Part model, mm, in its own coordinate system. Coordinates: 2 decimals unless noted, no trailing zeros. Order: outer loops, then holes, each group sorted by start corner. A loop starts at its lowest first (then second) coordinate and runs counter-clockwise, first axis right, second up.
Autodesk Inventor part; units mm, degrees
ref_plane "工作平面1" through (10, 22, 0) normal (-0.3882, -0.6516, -0.6516) x (0.8591, 0, -0.5118)
ref_plane "YZ Plane" through (0, 0, 0) normal (1, 0, 0) x (0, 1, 0)
ref_plane "XZ Plane" through (0, 0, 0) normal (0, 1, 0) x (-1, 0, 0)
sketch "草圖1" plane through (0, 0, 0) normal (0, 1, 0) x (-1, 0, 0)
  line L0 (0, 0) -> (-57, 0)
  line L1 (-57, 0) -> (-57, -38)
  line L2 (-57, -38) -> (0, -38)
  line L3 (0, -38) -> (0, 0)
  dimension "d0" = 57
  dimension "d1" = 38
extrude "擠出1" add sketch "草圖1" along normal mid plane 44
sketch "草圖2" plane through (0, 22, 0) normal (0, 1, 0) x (1, 0, 0)
  line L0 (0, 0) -> (57, 0)
  line L1 (10, 0) -> (57, 8)
  line L2 (57, 0) -> (57, 38)
  dimension "d4" = 10
  dimension "d5" = 30
extrude "擠出2" cut sketch "草圖2" against normal blind 60
sketch "草圖3" plane through (57, -22, -38) normal (1, 0, 0) x (0, 0, -1)
  line L0 (-30, 24) -> (-10, 44)
  line L1 (0, 44) -> (-38, 44)
  line L2 (-30, 44) -> (-30, 0)
  point P0 (-38, 22)
  point P1 (-30, 2)
  dimension "d8" = 20
  dimension "d9" = 20
ref_plane "工作平面1" through (10, 22, 0) normal (-0.3882, -0.6516, -0.6516) x (0.8591, 0, -0.5118)
sketch "草圖4" plane through (10, 22, 0) normal (-0.3882, -0.6516, -0.6516) x (0.8591, 0, -0.5118)
  line L0 (-15.1543, -12.3218) -> (93.717, -12.3218)
  line L1 (93.717, -12.3218) -> (93.717, 28.8166)
  line L2 (93.717, 28.8166) -> (-15.1543, 28.8166)
  line L3 (-15.1543, 28.8166) -> (-15.1543, -12.3218)
  point P0 (-8.591, 13.3523)
extrude "擠出3" cut sketch "草圖4" against normal blind 40
mirror "鏡射1" about plane through (0, 0, 0) normal (0, 1, 0) of "擠出3"
properties part number "52"
(1) Slice it at B-B, the plane x = 19. Give the cut face in (y, z).
(2) Drop flat-ended pins along their axis: pin 1 (12 mm diameter, centred on x = 28, y = -10, fed in from +Z); pin 2 (3 mm diameter, centred on x = 37, y = -5.5, fed in from +Z); pin 3 (1 mm diameter, centred on x = 32, z = -10, fed in from +Y). Give the stop position or say it passes through.
(3) Slice it at C-C, the plane z = -4.5. Give the cut face in (x, y), then the cut area to 3 significant figures.
(4) Slice it at A-A, the plane y = 1. Give the cut face in (x, z), then the cut area to 3 significant figures.
(5) Probe line 1 (Z direction, x = 53.5, y = 5.5); line 2 (X direction, y = 20.5, z = -24.5); line 3 (Z direction, x = 38, y = 13.5). List the from-to ranges inside material, lowest first.
Here are the results:
1. outline: (-22, -38) - (22, -38) - (22, -5.36) - (18.17, -1.53) - (-18.17, -1.53) - (-22, -5.36) - close
2. pin 1: stops at z = -2.04
2. pin 2: stops at z = -4.34
2. pin 3: stops at y = 19.47
3. outline: (0, -22) - (17.55, -22) - (36.44, -10.75) - (36.44, 10.75) - (17.55, 22) - (0, 22) - close
3. area: 1,390 mm2
4. outline: (0, -38) - (57, -38) - (57, -8) - (10, 0) - (0, 0) - close
4. area: 1,980 mm2
5. line 1: z = -38 to -9.42
5. line 2: x = 0 to 53.64
5. line 3: z = -38 to -8.18
